from build123d import *

# Parameters (mm, degrees)
SKIZZE1_R                            = 7
AUFSATZ_LINEAR_AUSTRAGEN1_DEPTH      = 3.5
SKIZZE2_R                            = 0.525
AUFSATZ_LINEAR_AUSTRAGEN2_DEPTH      = 1
KREISMUSTER1_COUNT                   = 4
SKIZZE3_R                            = 3
SCHNITT_LINEAR_AUSTRAGEN1_DEPTH      = 2
SCHNITT_LINEAR_AUSTRAGEN1_DEPTH_BACK = 2.65
SKIZZE4_R                            = 2
SCHNITT_LINEAR_AUSTRAGEN2_DEPTH      = 1.85
SKIZZE5_R                            = 2.25
SCHNITT_LINEAR_AUSTRAGEN3_DEPTH      = 2
KREISMUSTER2_COUNT                   = 4


with BuildPart() as part:
    # Skizze1 → Aufsatz-Linear austragen1 (new body)
    with BuildSketch(Plane.XY):
        Circle(SKIZZE1_R)
    extrude(amount=AUFSATZ_LINEAR_AUSTRAGEN1_DEPTH)

    # Skizze2 → Aufsatz-Linear austragen2 (add)
    with BuildSketch(Plane.XY.offset(3.5)):
        with Locations((0, 4)):
            Circle(SKIZZE2_R)
    aufsatz_linear_austragen2 = extrude(amount=AUFSATZ_LINEAR_AUSTRAGEN2_DEPTH)

    # Kreismuster1: Aufsatz-Linear austragen2 ×4 about axis
    kreismuster1_axis = Axis((0, 0, 0), (0, 0, 1))
    for i in range(1, KREISMUSTER1_COUNT):
        add(aufsatz_linear_austragen2.rotate(kreismuster1_axis, i * 360 / KREISMUSTER1_COUNT))

    # Skizze3 → Schnitt-Linear austragen1 (cut, two sides)
    with BuildSketch(Plane.XY.offset(3.5)) as schnitt_linear_austragen1_sk:
        Circle(SKIZZE3_R)
    extrude(amount=SCHNITT_LINEAR_AUSTRAGEN1_DEPTH, mode=Mode.SUBTRACT)
    extrude(schnitt_linear_austragen1_sk.sketch, amount=-SCHNITT_LINEAR_AUSTRAGEN1_DEPTH_BACK, mode=Mode.SUBTRACT)

    # Skizze4 → Schnitt-Linear austragen2 (cut, through all)
    with BuildSketch(Plane.XY.offset(0.85)):
        Circle(SKIZZE4_R)
    extrude(amount=-SCHNITT_LINEAR_AUSTRAGEN2_DEPTH, mode=Mode.SUBTRACT)

    # Skizze5 → Schnitt-Linear austragen3 (cut)
    with BuildSketch(Plane.XY.offset(3.5)):
        with Locations((-4.949747468, 4.949747468)):
            Circle(SKIZZE5_R)
    schnitt_linear_austragen3 = extrude(amount=-SCHNITT_LINEAR_AUSTRAGEN3_DEPTH, mode=Mode.SUBTRACT)

    # Kreismuster2: Schnitt-Linear austragen3 ×4 about axis
    kreismuster2_axis = Axis((0, 0, 0), (0, 0, 1))
    for i in range(1, KREISMUSTER2_COUNT):
        add(schnitt_linear_austragen3.rotate(kreismuster2_axis, i * 360 / KREISMUSTER2_COUNT), mode=Mode.SUBTRACT)


solid = part.part
For this review, take the finished solid that the model builds, in its own axes (mm). A direction names the side the tool comes from. Give positions to 0.01 mm unless a question says otherwise; leave off trailing zeros. Loops run counter-clockwise (first coordinate to the right, second up) from the corner with the lowest first, then second, coordinate; pieces in that order, holes last.
Item 1: Take a section at C-C, the plane z = 2.4. State the section outline as (x, y) points.
Item 2: Tool access review of faces 4 (the cylindrical face through (-3, 0, 2)), 5 (the flat face through (-4, 0, 4.5)): name each direction out of +Z, -Z, +X, -X, +Y, -Y from which nothing blocks a thin tool from reaching the whole face with its end or side.
Item 3: Insertion check: pin 1 (6.5 mm diameter, centred on x = 0, y = 0, fed in from -Z); pin 2 (3 mm diameter, centred on x = -1, y = -0.5, fed in from +Z); pin 3 (4 mm diameter, centred on x = -4, y = 3.5, fed in from +Z); pin 4 (3 mm diameter, centred on x = 5, y = 4.5, fed in from +Z). Each pin has a flat end and moves straight along its axis. Give the tip position at first contact, or say it passes through.
Item 4: Draft analysis for pull direction Y (two halves, no side actions). For faces 1 (the flat face through (4, 0, 4.5)), 2 (the cylindrical face through (6.466, -2.681, 1.337)), 3 (the cylindrical face through (-3.39, 3.33, 2.51)), state which applies: +Y half, -Y half, draft (parallel to the pull), parting line (faces both ways), or undercut.
Item 5: For line 1 along Y through (x, z) = (0, 0.45); line 2 along Z through (x, y) = (2, 6); line 3 along Y through (x, z) = (0, 1.8), list the stretches that pass through material, from the lowest coordinate up.
Item 6: Take a section at D-D, the plane x = -4.25. State the section outline as (y, z) points, and give its area (3 significant figures).
Item 7: Take a section at A-A, the plane x = 0. State the section outline as (y, z) points (3 decimals), and give its area (3 significant figures).
Item 8: Take a section at B-B, the plane y = 0.25. State the section outline as (x, z) points, and give its area (3 significant figures).
Calculated:
1. outline: (-6.26, -3.12) arc R2.25 cw to (-3.12, -6.26) arc R7 ccw to (3.12, -6.26) arc R2.25 cw to (6.26, -3.12) arc R7 ccw to (6.26, 3.12) arc R2.25 cw to (3.12, 6.26) arc R7 ccw to (-3.12, 6.26) arc R2.25 cw to (-6.26, 3.12) arc R7 ccw to start; hole circle Ø6 at (0, 0)
2. face 4: +Z
2. face 5: +Z, +X, -X, +Y, -Y
3. pin 1: stops at z = 0
3. pin 2: stops at z = 0.85
3. pin 3: stops at z = 3.5
3. pin 4: stops at z = 1.5
4. face 1: draft
4. face 2: parting line
4. face 3: undercut
5. line 1: y = -7 to -2, 2 to 7
5. line 2: z = 0 to 3.5
5. line 3: y = -7 to -3, 3 to 7
6. outline: (-5.56, 0) - (5.56, 0) - (5.56, 1.5) - (2.81, 1.5) - (2.81, 3.5) - (0.46, 3.5) - (0.46, 4.5) - (-0.46, 4.5) - (-0.46, 3.5) - (-2.81, 3.5) - (-2.81, 1.5) - (-5.56, 1.5) - close
6. area: 28.9 mm2
7. outline: (-7, 0) - (-2, 0) - (-2, 0.85) - (-3, 0.85) - (-3, 3.5) - (-3.475, 3.5) - (-3.475, 4.5) - (-4.525, 4.5) - (-4.525, 3.5) - (-7, 3.5) - close; (2, 0) - (7, 0) - (7, 3.5) - (4.525, 3.5) - (4.525, 4.5) - (3.475, 4.5) - (3.475, 3.5) - (3, 3.5) - (3, 0.85) - (2, 0.85) - close
7. area: 31.8 mm2
8. outline: (-7, 0) - (-1.98, 0) - (-1.98, 0.85) - (-2.99, 0.85) - (-2.99, 3.5) - (-3.54, 3.5) - (-3.54, 4.5) - (-4.46, 4.5) - (-4.46, 3.5) - (-7, 3.5) - close; (1.98, 0) - (7, 0) - (7, 3.5) - (4.46, 3.5) - (4.46, 4.5) - (3.54, 4.5) - (3.54, 3.5) - (2.99, 3.5) - (2.99, 0.85) - (1.98, 0.85) - close
8. area: 31.6 mm2
